CAD build for the part. Positions are in the model's coordinates, mm. A direction names the side the tool comes from. Give positions to 0.01 mm unless a question says otherwise; leave off trailing zeros. Write each loop counter-clockwise with the first axis right and the second up, starting at its lowest first coordinate (ties: lowest second). Pieces come first, ordered by that corner, then holes. Notation, with made-up numbers: (-24.5, 41) - (28.5, 41) arc R9 cw to (28.5, 50) - close; hole circle Ø1 at (7, 32). An arc over 180 degrees is marked (long way). Put each result on its own line as item: value. Start each with the question number.
1. Drop flat-ended pins along their axis: pin 1 (9 mm diameter, centred on x = -30, y = 35, fed in from +Z); pin 2 (20 mm diameter, centred on x = 3, y = 8.5, fed in from +Z); pin 3 (18 mm diameter, centred on x = 7.5, y = -11.5, fed in from +Z). Give the stop position or say it passes through.
2. Tool access for faces 1 (the flat face through (6, -20, 3.5)), 2 (the cylindrical face through (-41.07, 46, 2.54)): list every direction of +Z, -Z, +X, -X, +Y, -Y with a clear straight run to the whole face (end or side of a thin tool).
3. Cut at C-C on x = 15. List the corners of the cut face in (y, z).
4. Cut at A-A on y = 0. List the corners of the cut face in (x, z), and give its area (3 significant figures).
5. Cut at B-B on y = -37. List the corners of the cut face in (x, z), and give its area (3 significant figures).
6. Wall check: line 1 (Y direction, x = -30, z = 2.65); line 2 (X direction, y = -31, z = 0.8); line 3 (Y direction, x = 0, z = 2.9). Give the ranges that are in metal, low to high.
7. Mould opens along Y. For faces 3 (the cylindrical face through (41, 46.07, 2.54)), 4 (the cylindrical face through (-4.336, -19.524, 2.993)), 5 (the flat face through (-42.5, -1, 2)), 6 (the flat face through (4, -4, 2.5)) say: +Y half, -Y half, draft (parallel to the pull), parting line (faces both ways), or undercut.
from build123d import *

# Parameters (mm, degrees)
F0_W     = 85
F0_H     = 95
F0_R     = 5
F0_R_2   = 30
F1_DEPTH = 5
F0_R_3   = 20
F2_DEPTH = 2.5
F3_DEPTH = 3.5
F4_R     = 5


with BuildPart() as f1:
    # F0 (on Top) → F1 (new body)
    with BuildSketch(Plane.XY):
        Rectangle(F0_W, F0_H)
        with Locations((-30, -35)):
            Circle(F0_R, mode=Mode.SUBTRACT)
        with Locations((30, -35)):
            Circle(F0_R, mode=Mode.SUBTRACT)
        with Locations((-30, 35)):
            Circle(F0_R, mode=Mode.SUBTRACT)
        Circle(F0_R_2, mode=Mode.SUBTRACT)
        with Locations((30, 35)):
            Circle(F0_R, mode=Mode.SUBTRACT)
    extrude(amount=F1_DEPTH)

    # F0 (on Top) → F2 (join)
    with BuildSketch(Plane.XY):
        Circle(F0_R_2)
        Circle(F0_R_3, mode=Mode.SUBTRACT)
        Circle(F0_R_3)
        Circle(F0_R, mode=Mode.SUBTRACT)
    extrude(amount=F2_DEPTH)

    # F0 (on Top) → F3 (join)
    with BuildSketch(Plane.XY):
        Circle(F0_R_2)
        Circle(F0_R_3, mode=Mode.SUBTRACT)
    extrude(amount=F3_DEPTH)

    # F4
    f4_edges = [f1.edges().sort_by_distance(p)[0] for p in [
        (-42.5, -47.5, 2.5),
        (42.5, -47.5, 2.5),
        (42.5, 47.5, 2.5),
        (-42.5, 47.5, 2.5),
    ]]
    fillet(f4_edges, radius=F4_R)


solid = f1.part
Report:
1. pin 1: passes through
1. pin 2: stops at z = 2.5
1. pin 3: stops at z = 3.5
2. face 1: +Z
2. face 2: +Z, -Z, -X, +Y
3. outline: (-47.5, 0) - (47.5, 0) - (47.5, 5) - (25.98, 5) - (25.98, 3.5) - (13.23, 3.5) - (13.23, 2.5) - (-13.23, 2.5) - (-13.23, 3.5) - (-25.98, 3.5) - (-25.98, 5) - (-47.5, 5) - close
4. outline: (-42.5, 0) - (-5, 0) - (-5, 2.5) - (-20, 2.5) - (-20, 3.5) - (-30, 3.5) - (-30, 5) - (-42.5, 5) - close; (5, 0) - (42.5, 0) - (42.5, 5) - (30, 5) - (30, 3.5) - (20, 3.5) - (20, 2.5) - (5, 2.5) - close
4. area: 270 mm²
5. outline: (-42.5, 0) - (-34.58, 0) - (-34.58, 5) - (-42.5, 5) - close; (-25.42, 0) - (25.42, 0) - (25.42, 5) - (-25.42, 5) - close; (34.58, 0) - (42.5, 0) - (42.5, 5) - (34.58, 5) - close
5. area: 333 mm²
6. line 1: y = -47.5 to -40, -30 to 30, 40 to 47.5
6. line 2: x = -42.5 to -33, -27 to 27, 33 to 42.5
6. line 3: y = -47.5 to -20, 20 to 47.5
7. face 3: +Y half
7. face 4: undercut
7. face 5: draft
7. face 6: undercut
